Check sheet for the modelled part. Datum: model origin and axes. Units: mm. A direction names the side the tool comes from. Coordinates: 2 decimals unless noted, no trailing zeros. Loops run counter-clockwise (first coordinate to the right, second up) from the corner with the lowest first, then second, coordinate; pieces in that order, holes last. Notation, with made-up numbers: M -23.5,5.5 L 1.5,5.5 A16 ccw 1.5,12.5 Z; hole C 79.25,51 d6. An arc over 180 degrees is marked long. Return JSON: item names as keys, results as strings.
from build123d import *

# Parameters (mm, degrees)
SKETCH_1_R      = 37.5
SKETCH_1_R_2    = 3.25
SKETCH_1_R_3    = 2.75
EXTRUDE_1_DEPTH = 5


with BuildPart() as part:
    # 草图1 → 凸台-拉伸1 (new body)
    with BuildSketch(Plane.XY):
        Polygon((0, 0), (-135, 0), (-135, 30), (-165, 30), (-165, 165), (0, 165), align=None)
        with Locations((-67.5, 97.5)):
            Circle(SKETCH_1_R, mode=Mode.SUBTRACT)
        with Locations((-102.25, 132.25)):
            Circle(SKETCH_1_R_2, mode=Mode.SUBTRACT)
        with Locations((-32.75, 132.25)):
            Circle(SKETCH_1_R_2, mode=Mode.SUBTRACT)
        with Locations((-32.75, 62.75)):
            Circle(SKETCH_1_R_2, mode=Mode.SUBTRACT)
        with Locations((-102.25, 62.75)):
            Circle(SKETCH_1_R_2, mode=Mode.SUBTRACT)
        with Locations((-150, 147.5)):
            Circle(SKETCH_1_R_3, mode=Mode.SUBTRACT)
        with Locations((-150, 97.5)):
            Circle(SKETCH_1_R_3, mode=Mode.SUBTRACT)
        with Locations((-67.5, 15)):
            Circle(SKETCH_1_R_3, mode=Mode.SUBTRACT)
        with Locations((-17.5, 15)):
            Circle(SKETCH_1_R_3, mode=Mode.SUBTRACT)
        with Locations((-117.5, 15)):
            Circle(SKETCH_1_R_3, mode=Mode.SUBTRACT)
        with Locations((-150, 47.5)):
            Circle(SKETCH_1_R_3, mode=Mode.SUBTRACT)
    extrude(amount=EXTRUDE_1_DEPTH)


solid = part.part
1) Section check C-C on x = -17.5. Record the cut outline in (y, z), then the cut area to 4 significant figures.
Answers:
{"outline": "M 0,0 L 12.25,0 L 12.25,5 L 0,5 Z; M 17.75,0 L 165,0 L 165,5 L 17.75,5 Z", "area": "797.5 mm²"}
2) Section check D-D on y = 147.5. Record the cut outline in (x, z), then the cut area to 4 significant figures.
Answers:
{"outline": "M -165,0 L -152.75,0 L -152.75,5 L -165,5 Z; M -147.25,0 L 0,0 L 0,5 L -147.25,5 Z", "area": "797.5 mm²"}
3) Section check A-A on z = 2.3. Count the separate pieces of the cut face and the enclosed holes in it, then the cut area to 3 significant figures.
Answers:
{"separate pieces": "1", "enclosed holes": "11", "area": "21,600 mm²"}
4) Section check B-B on y = 97.5. Record the cut outline in (x, z).
Answers:
{"outline": "M -165,0 L -152.75,0 L -152.75,5 L -165,5 Z; M -147.25,0 L -105,0 L -105,5 L -147.25,5 Z; M -30,0 L 0,0 L 0,5 L -30,5 Z"}
5) Go/stop test with flat-tipped pins: pin 1 Ø8.5 at (x, y) = (-102.25, 132.25) entering from -Z; pin 2 Ø3.5 at (x, y) = (-150, 147.5) entering from +Z. Record where each tip stops, or that it passes through.
Answers:
{"pin 1": "z = 0", "pin 2": "through"}
6) Draft check along Y on faces 1 (the face through (-105.497, 62.893, 2.465)), 2 (the face through (-67, 0, 2)), 3 (the face through (-99.7, 65.3, 0)). Enter one of: +Y half, -Y half, draft (parallel to the pull), parting line (faces both ways), or undercut.
Answers:
{"face 1": "undercut", "face 2": "-Y half", "face 3": "draft"}
7) Scan lines: line 1 along X through (y, z) = (132.25, 1.35); line 2 along Y through (x, z) = (-66.5, 3.3); line 3 along Y through (x, z) = (-102, 1.7). Record each from-to range of solid material in increasing order. Write a range as [from, to].
Answers:
{"line 1": "[-165, -105.5], [-99, -81.6], [-53.4, -36], [-29.5, 0]", "line 2": "[0, 12.44], [17.56, 60.01], [134.99, 165]", "line 3": "[0, 59.51], [65.99, 82.8], [112.2, 129.01], [135.49, 165]"}
8) Set-up check for faces 4 (the face through (-147.46, 146.45, 2.46)), 5 (the face through (-135, 15, 2)): record each of +Z, -Z, +X, -X, +Y, -Y from which the full face is reachable in a straight line by a thin tool's end or side.
Answers:
{"face 4": "+Z, -Z", "face 5": "+Z, -Z, -X, -Y"}
